Read the model definition and answer for the solid it produces. Units are mm, in the model's axes. Give positions to 0.01 mm unless a question says otherwise; leave off trailing zeros. Order: outer loops, then holes, each group sorted by start corner. A loop starts at its lowest first (then second) coordinate and runs counter-clockwise, first axis right, second up.
```python
from build123d import *

# Parameters (mm, degrees)
BOSS_EXTRUDE1_DEPTH     = 7.62
SKETCH2_W               = 85.677392152
SKETCH2_H               = 16.256
CUT_EXTRUDE1_DEPTH      = 1
CUT_EXTRUDE1_DEPTH_BACK = 8.62
FILLET1_R               = 5.08
SKETCH3_W               = 10.16
SKETCH3_H               = 7.62
CUT_EXTRUDE2_DEPTH      = 8.62
SKETCH4_W               = 25.4
SKETCH4_H               = 10.16
CUT_EXTRUDE3_DEPTH      = 8.62
SKETCH5_W               = 7.62
SKETCH5_H               = 15.24
CUT_EXTRUDE5_DEPTH      = 8.62


with BuildPart() as part:
    # Sketch1 → Boss-Extrude1 (new body)
    with BuildSketch(Plane(origin=(0, 0, 0), x_dir=(1, 0, 0), z_dir=(0, 1, 0))):
        with BuildLine():
            Line((-88.9, 0), (-88.9, 76.2))
            ThreePointArc((-88.9, 76.2), (0, 165.1), (88.9, 76.2))
            Line((88.9, 76.2), (88.9, 0))
            ThreePointArc((88.9, 0), (0, -88.9), (-88.9, 0))
        make_face()
    extrude(amount=BOSS_EXTRUDE1_DEPTH)

    # Sketch2 → Cut-Extrude1 (cut, two sides)
    with BuildSketch(Plane(origin=(0, 7.62, 0), x_dir=(1, 0, 0), z_dir=(0, 1, 0))) as cut_extrude1_sk:
        with Locations((0, -58.235236409)):
            Rectangle(SKETCH2_W, SKETCH2_H)
        with Locations((0, 134.435236409)):
            Rectangle(SKETCH2_W, SKETCH2_H)
    extrude(amount=CUT_EXTRUDE1_DEPTH, mode=Mode.SUBTRACT)
    extrude(cut_extrude1_sk.sketch, amount=-CUT_EXTRUDE1_DEPTH_BACK, mode=Mode.SUBTRACT)

    # Fillet1
    fillet1_edges = [part.edges().sort_by_distance(p)[0] for p in [
        (-42.838696076, 3.81, 66.363236409),
        (-42.838696076, 3.81, 50.107236409),
        (42.838696076, 3.81, 50.107236409),
        (42.838696076, 3.81, 66.363236409),
        (-42.838696076, 3.81, -126.307236409),
        (-42.838696076, 3.81, -142.563236409),
        (42.838696076, 3.81, -142.563236409),
        (42.838696076, 3.81, -126.307236409),
    ]]
    fillet(fillet1_edges, radius=FILLET1_R)

    # Sketch3 → Cut-Extrude2 (cut, through all)
    with BuildSketch(Plane(origin=(0, 7.62, 0), x_dir=(1, 0, 0), z_dir=(0, 1, 0))):
        with Locations((10.922, 87.445236409)):
            Rectangle(SKETCH3_W, SKETCH3_H)
        with Locations((-10.922, 87.445236409)):
            Rectangle(SKETCH3_W, SKETCH3_H)
        with Locations((10.922, 120.973236409)):
            Rectangle(SKETCH3_W, SKETCH3_H)
        with Locations((-10.922, 120.973236409)):
            Rectangle(SKETCH3_W, SKETCH3_H)
        with Locations((-10.922, -11.245236409)):
            Rectangle(SKETCH3_W, SKETCH3_H)
        with Locations((10.922, -11.245236409)):
            Rectangle(SKETCH3_W, SKETCH3_H)
        with Locations((-10.922, -44.773236409)):
            Rectangle(SKETCH3_W, SKETCH3_H)
        with Locations((10.922, -44.773236409)):
            Rectangle(SKETCH3_W, SKETCH3_H)
    extrude(amount=-CUT_EXTRUDE2_DEPTH, mode=Mode.SUBTRACT)

    # Sketch4 → Cut-Extrude3 (cut, through all)
    with BuildSketch(Plane(origin=(0, 7.62, 0), x_dir=(1, 0, 0), z_dir=(0, 1, 0))):
        with Locations((0, 67.537940424)):
            Rectangle(SKETCH4_W, SKETCH4_H)
        with Locations((0, 8.662059576)):
            Rectangle(SKETCH4_W, SKETCH4_H)
    extrude(amount=-CUT_EXTRUDE3_DEPTH, mode=Mode.SUBTRACT)

    # Sketch5 → Cut-Extrude5 (cut, through all)
    with BuildSketch(Plane(origin=(0, 7.62, 0), x_dir=(1, 0, 0), z_dir=(0, 1, 0))):
        with Locations((80.01, -11.43)):
            Rectangle(SKETCH5_W, SKETCH5_H)
        with Locations((-80.01, -11.43)):
            Rectangle(SKETCH5_W, SKETCH5_H)
        with Locations((-80.01, 87.63)):
            Rectangle(SKETCH5_W, SKETCH5_H)
        with Locations((80.01, 87.63)):
            Rectangle(SKETCH5_W, SKETCH5_H)
    extrude(amount=-CUT_EXTRUDE5_DEPTH, mode=Mode.SUBTRACT)


solid = part.part
```
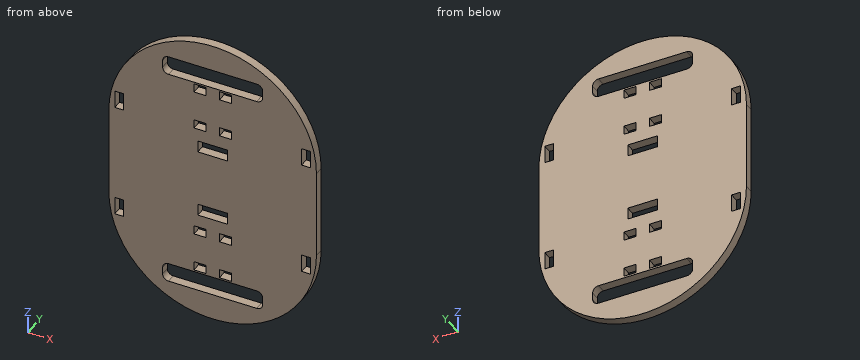
1) Given pin 1 (1.5 mm diameter, centred on y = 4.5, z = -124, fed in from -X); pin 2 (8 mm diameter, centred on x = -47, z = -125.5, fed in from -Y); pin 3 (2.5 mm diameter, centred on x = 11, y = 3, fed in from +Z); pin 4 (2 mm diameter, centred on y = 1, z = -95, fed in from +X), each flat-ended and moving along its own axis, determine where each tip first touches the part or whether it passes through.
Final values:
pin 1: stops at x = -75.43
pin 2: stops at y = 0
pin 3: stops at z = 88.36
pin 4: stops at x = 87.1
2) The part is cut by section A-A on x = 0. Determine the outline of the cut face in (y, z), and give its area (3 significant figures).
Final values:
outline: (0, -165.1) - (7.62, -165.1) - (7.62, -142.56) - (0, -142.56) - close; (0, -126.31) - (7.62, -126.31) - (7.62, -72.62) - (0, -72.62) - close; (0, -62.46) - (7.62, -62.46) - (7.62, -13.74) - (0, -13.74) - close; (0, -3.58) - (7.62, -3.58) - (7.62, 50.11) - (0, 50.11) - close; (0, 66.36) - (7.62, 66.36) - (7.62, 88.9) - (0, 88.9) - close
area: 1,530 mm2
3) The part is cut by section D-D on x = 33. Determine the outline of the cut face in (y, z).
Final values:
outline: (0, -158.75) - (7.62, -158.75) - (7.62, -142.56) - (0, -142.56) - close; (0, -126.31) - (7.62, -126.31) - (7.62, 50.11) - (0, 50.11) - close; (0, 66.36) - (7.62, 66.36) - (7.62, 82.55) - (0, 82.55) - close
4) The part is cut by section C-C on y = 2.75. Count the separate pieces of the cut face and the enclosed holes in it, and give its area (3 significant figures).
Final values:
separate pieces: 1
enclosed holes: 16
area: 34,000 mm2
5) Consider L1, parallel to X at y = 5.75, z = -11; L2, parallel to Z at x = 26, y = 2.5; L3, parallel to X at y = 1.75, z = 6. Determine where each line is inside the solid, lowest interval first.
Final values:
L1: x = -88.9 to -12.7, 12.7 to 88.9
L2: z = -161.21 to -142.56, -126.31 to 50.11, 66.36 to 85.01
L3: x = -88.7 to -83.82, -76.2 to 76.2, 83.82 to 88.7
6) The part is cut by section B-B on z = -120. Determine the outline of the cut face in (x, y).
Final values:
outline: (-77.36, 0) - (-16, 0) - (-16, 7.62) - (-77.36, 7.62) - close; (-5.84, 0) - (5.84, 0) - (5.84, 7.62) - (-5.84, 7.62) - close; (16, 0) - (77.36, 0) - (77.36, 7.62) - (16, 7.62) - close
